```python
from build123d import *

# Parameters (mm, degrees)
BOSS_EXTRUDE1_DEPTH = 6
SKETCH2_R           = 5
BOSS_EXTRUDE2_DEPTH = 35
FILLET1_R           = 1
SKETCH3_W           = 16
SKETCH3_H           = 32
BOSS_EXTRUDE3_DEPTH = 1.5
CUT_EXTRUDE1_REACH  = 69.891
SKETCH4_R           = 3


with BuildPart() as part:
    # Sketch1 → Boss-Extrude1 (new, symmetric)
    with BuildSketch(Plane.XY):
        Polygon((-6, -14), (-6, 14), (6, 14), (6, -14), (4, -14), (4, -16), (8, -16), (8, 16), (-8, 16), (-8, -16), (-4, -16), (-4, -14), align=None)
    extrude(amount=BOSS_EXTRUDE1_DEPTH, both=True)

    # Sketch2 → Boss-Extrude2 (add)
    with BuildSketch(Plane(origin=(0, 16, 0), x_dir=(1, 0, 0), z_dir=(0, 1, 0))):
        with Locations(Location((0, 0, 0), (0, 0, 270))):
            Circle(SKETCH2_R)
    extrude(amount=BOSS_EXTRUDE2_DEPTH)

    # Fillet1
    fillet1_edges = [part.edges().sort_by_distance(p)[0] for p in [
        (0, 16, -5),
    ]]
    fillet(fillet1_edges, radius=FILLET1_R - 0.0001)  # a hair under: the kernel refuses the full size

    # Sketch3 → Boss-Extrude3 (add)
    with BuildSketch(Plane.XY.offset(6)):
        Rectangle(SKETCH3_W, SKETCH3_H)
    extrude(amount=BOSS_EXTRUDE3_DEPTH)

    # Sketch4 → Cut-Extrude1 (cut, up to next)
    with BuildSketch(Plane(origin=(0, 51, 0), x_dir=(1, 0, 0), z_dir=(0, 1, 0)), mode=Mode.PRIVATE) as cut_extrude1_sk1:
        with Locations(Location((0, 0, 0), (0, 0, 270))):
            Circle(SKETCH4_R)
    cut_extrude1_tool1 = extrude(cut_extrude1_sk1.sketch, amount=-CUT_EXTRUDE1_REACH, mode=Mode.PRIVATE) & part.part
    add(cut_extrude1_tool1.solids().sort_by_distance((0, 51, 0))[0], mode=Mode.SUBTRACT)


solid = part.part
```
Could you check a few things on this model? Use its own coordinates, in mm. A direction names the side the tool comes from. Round coordinates to 2 decimals unless told otherwise and drop trailing zeros. Loops run counter-clockwise (first coordinate to the right, second up) from the corner with the lowest first, then second, coordinate; pieces in that order, holes last. Notation, with made-up numbers: (8.25, 58) - (21.25, 58) arc R19 cw to (21.25, 84) - close; hole circle Ø3 at (6.5, 10). An arc over 180 degrees is marked (long way). Answer in a Markdown table with one row per item. Add a question column.
(1) For faces 1 (the face through (-4.88, 33.76, -1.08)), 2 (the face through (-4, -15, 0)), 3 (the face through (6, 0, 0)), which set-ups out of +Z, -Z, +X, -X, +Y, -Y let a thin tool reach every point of the face, with its end or its side?
(2) If we section it at A-A (z = 0): Please give me the cut outline in (x, y), plus the area to 3 significant figures.
(3) If we section it at B-B (y = -10.5): Please give me the cut outline in (x, z), plus the area to 3 significant figures.
(4) I need wall thicknesses on line 1 along X through (y, z) = (34, 0); line 2 along X through (y, z) = (11.5, 0); line 3 along Y through (x, z) = (5.75, -4.25). Which ranges of each line are inside material? Lowest first, please.
(5) If we mould it in two halves opening along Y, with no side actions, what happens to faces 4 (the face through (4, -15, 0)), 5 (the face through (-4, 16, 5)), 6 (the face through (-6, 0, 0)), 7 (the face through (0, -16, 7))? For each: pulls with the +Y half, pulls with the -Y half, needs draft (parallel to the pull), parting line crosses it, or undercut.
(6) If we section it at D-D (y = 45): Please give me the cut outline in (x, z).
(7) I'm going to push flat-ended pins straight in: pin 1 (5 mm diameter, centred on x = -2, y = 30, fed in from -Z); pin 2 (2 mm diameter, centred on y = 26, z = 2, fed in from +X); pin 3 (4 mm diameter, centred on y = 26, z = 5, fed in from +X). Where does each tip first touch, or does it pass through?
Model answer:
| question | item | result |
|---|---|---|
| 1 | face 1 | +Y |
| 1 | face 2 | -Z, -Y |
| 1 | face 3 | -Z |
| 2 | outline | (-8, -16) - (-4, -16) - (-4, -14) - (-6, -14) - (-6, 14) - (-3, 14) - (-3, 51) - (-5, 51) - (-5, 17) arc R1 cw to (-6, 16) - (-8, 16) - close; (3, 14) - (6, 14) - (6, -14) - (4, -14) - (4, -16) - (8, -16) - (8, 16) - (6, 16) arc R1 cw to (5, 17) - (5, 51) - (3, 51) - close |
| 2 | area | 288 mm² |
| 3 | outline | (-8, -6) - (-6, -6) - (-6, 6) - (6, 6) - (6, -6) - (8, -6) - (8, 7.5) - (-8, 7.5) - close |
| 3 | area | 72.0 mm² |
| 4 | line 1 | x = -5 to -3, 3 to 5 |
| 4 | line 2 | x = -8 to -6, 6 to 8 |
| 4 | line 3 | y = -16 to -14, 14 to 16 |
| 5 | face 4 | needs draft |
| 5 | face 5 | pulls with the +Y half |
| 5 | face 6 | undercut |
| 5 | face 7 | pulls with the -Y half |
| 6 | outline | circle Ø10 at (0, 0); hole circle Ø6 at (0, 0) |
| 7 | pin 1 | stops at z = -5 |
| 7 | pin 2 | stops at x = 4.9 |
| 7 | pin 3 | stops at x = 4 |
